For this review, take the finished solid that the model builds, in its own axes (mm). Face numbers are marked on the shaded views. A direction names the side the tool comes from. Give positions to 0.01 mm unless a question says otherwise; leave off trailing zeros. Write each loop counter-clockwise with the first axis right and the second up, starting at its lowest first coordinate (ties: lowest second). Pieces come first, ordered by that corner, then holes.
1) We need section B-B on x = 21.5. Give the boundary of the cut face in (y, z), and give its area (3 significant figures).
2) For P1, Ø1.5, axis at x = 5, z = 4, coming from the -Y side; P2, Ø2, axis at x = 21.5, z = 17.5, coming from the +Y side; P3, Ø7.5, axis at y = -0.5, z = 25, coming from the -X side; P4, Ø2.5, axis at x = 22.5, y = 2.5, coming from the +Z side, all flat-tipped, find the tip position at first contact; note any pin that passes through.
3) Machinability: for the marked faces 1 and 2, which of the approach directions +Z, -Z, +X, -X, +Y, -Y give a long, thin tool a straight path to every point of the face, cutting with its end or side? Answer none if there is none.
4) We need section A-A on x = 0. Give the boundary of the cut face in (y, z).
5) Draft analysis for pull direction X (two halves, no side actions). For the marked faces 3, 4 and 5, state which applies: pulls with the +X half, pulls with the -X half, needs draft (parallel to the pull), parting line crosses it, or undercut.
6) We need section C-C on z = 32.5. Give the boundary of the cut face in (x, y), and give its area (3 significant figures).
7) We need section D-D on z = 17.5. Give the number of separate pieces and of enclosed holes in the cut face, and give its area (3 significant figures).
8) Wall thickness on line 1 along X through (y, z) = (1.5, 18); line 2 along X through (y, z) = (6.75, 17.5); line 3 along Z through (x, y) = (21.5, 1.65): over which ranges is each line inside the solid? List them lowest first.
from build123d import *

# Parameters (mm, degrees)
BOSS_EXTRUDE1_DEPTH  = 35
SKETCH3_W            = 7
SKETCH3_H            = 7
BOSS_EXTRUDE2_DEPTH  = 3
FILLET1_R            = 2
FILLET2_R            = 0.5
M2_CLEARANCE_HOLE1_D = 2.6
FILLET3_R            = 0.5
FILLET4_R            = 2
FILLET5_R            = 10
SKETCH8_W            = 20
SKETCH8_H            = 2
BOSS_EXTRUDE4_DEPTH  = 20
M4_CLEARANCE_HOLE1_D = 4.8
FILLET6_R            = 3
FILLET7_R            = 1


with BuildPart() as part:
    # Sketch1 → Boss-Extrude1 (new body)
    with BuildSketch(Plane.XY):
        with BuildLine():
            Line((13.479150567, 0.75), (17.5, 0.75))
            Line((17.5, 0.75), (17.5, 17.5))
            Line((17.5, 17.5), (-17.5, 17.5))
            Line((-17.5, 17.5), (-17.5, -17.5))
            Line((-17.5, -17.5), (17.5, -17.5))
            Line((17.5, -17.5), (17.5, -0.75))
            Line((17.5, -0.75), (13.479150567, -0.75))
            ThreePointArc((13.479150567, -0.75), (-13.5, 0), (13.479150567, 0.75))
        make_face()
    extrude(amount=BOSS_EXTRUDE1_DEPTH)

    # Sketch3 → Boss-Extrude2 (add)
    with BuildSketch(Plane.XZ.offset(-0.75)):
        with Locations((21, 17.5)):
            Rectangle(SKETCH3_W, SKETCH3_H)
    boss_extrude2 = extrude(amount=-BOSS_EXTRUDE2_DEPTH)

    # Fillet1
    fillet1_edges = [part.edges().sort_by_distance(p)[0] for p in [
        (17.5, 3.75, 17.5),
    ]]
    fillet(fillet1_edges, radius=FILLET1_R)

    # Fillet2
    fillet2_edges = [part.edges().sort_by_distance(p)[0] for p in [
        (24.5, 3.75, 17.5),
    ]]
    fillet(fillet2_edges, radius=FILLET2_R)

    # M2 Clearance Hole1 (through all)
    with Locations(Plane(origin=(0, 3.75, 0), x_dir=(1, 0, 0), z_dir=(0, 1, 0))):
        with Locations((21.5, -17.5)):
            m2_clearance_hole1 = Hole(M2_CLEARANCE_HOLE1_D / 2)

    # Mirror3: Boss-Extrude2 across plane
    add(boss_extrude2.mirror(Plane.ZX))

    # Mirror5: M2 Clearance Hole1 across plane
    add(m2_clearance_hole1.mirror(Plane.ZX), mode=Mode.SUBTRACT)

    # Fillet3
    fillet3_edges = [part.edges().sort_by_distance(p)[0] for p in [
        (24.5, -3.75, 17.5),
    ]]
    fillet(fillet3_edges, radius=FILLET3_R)

    # Fillet4
    fillet4_edges = [part.edges().sort_by_distance(p)[0] for p in [
        (17.5, -3.75, 17.5),
    ]]
    fillet(fillet4_edges, radius=FILLET4_R)

    # Fillet5
    # the kernel refuses this fillet: 10 mm, written as the material it takes off along each edge
    with BuildSketch(Plane(origin=(-42.5, -17.5, 0), x_dir=(0, 0, 1), z_dir=(1, 0, 0)), Plane(origin=(17.5, -17.5, -25), x_dir=(-1, 0, 0), z_dir=(0, 0, 1)), Plane(origin=(42.5, 17.5, 35), x_dir=(0, -1, 0), z_dir=(-1, 0, 0)), Plane(origin=(42.5, 17.5, 0), x_dir=(0, 0, 1), z_dir=(-1, 0, 0)), Plane(origin=(-42.5, -17.5, 35), x_dir=(0, 1, 0), z_dir=(1, 0, 0))) as fillet5_piece_1:
        with BuildLine():
            CenterArc((FILLET5_R, -FILLET5_R), FILLET5_R, 90, 90)
            Line((0, -FILLET5_R), (0, 0))
            Line((0, 0), (FILLET5_R, 0))
        make_face()
    extrude(amount=85, mode=Mode.SUBTRACT)
    with BuildSketch(Plane(origin=(-17.5, 17.5, -25), x_dir=(0, -1, 0), z_dir=(0, 0, 1)), Plane(origin=(17.5, 17.5, -25), x_dir=(-1, 0, 0), z_dir=(0, 0, 1)), Plane(origin=(-17.5, -17.5, -25), x_dir=(1, 0, 0), z_dir=(0, 0, 1))) as fillet5_piece_2:
        with BuildLine():
            CenterArc((FILLET5_R, FILLET5_R), FILLET5_R, 180, 90)
            Line((0, FILLET5_R), (0, 0))
            Line((0, 0), (FILLET5_R, 0))
        make_face()
    extrude(amount=85, mode=Mode.SUBTRACT)

    # Sketch8 → Boss-Extrude4 (add)
    with BuildSketch(Plane.ZY.offset(17.5)):
        with Locations((17.5, 6.5)):
            Rectangle(SKETCH8_W, SKETCH8_H)
    extrude(amount=BOSS_EXTRUDE4_DEPTH)

    # M4 Clearance Hole1 (through all)
    with Locations(Plane(origin=(0, 7.5, 0), x_dir=(1, 0, 0), z_dir=(0, 1, 0))):
        with Locations((-29.5, -17.5)):
            Hole(M4_CLEARANCE_HOLE1_D / 2)

    # Fillet6
    fillet6_edges = [part.edges().sort_by_distance(p)[0] for p in [
        (-17.5, 5.5, 17.5),
        (-17.5, 7.5, 17.5),
    ]]
    fillet(fillet6_edges, radius=FILLET6_R)

    # Fillet7
    fillet7_edges = [part.edges().sort_by_distance(p)[0] for p in [
        (-37.5, 6.5, 7.5),
        (-37.5, 6.5, 27.5),
    ]]
    fillet(fillet7_edges, radius=FILLET7_R)


solid = part.part
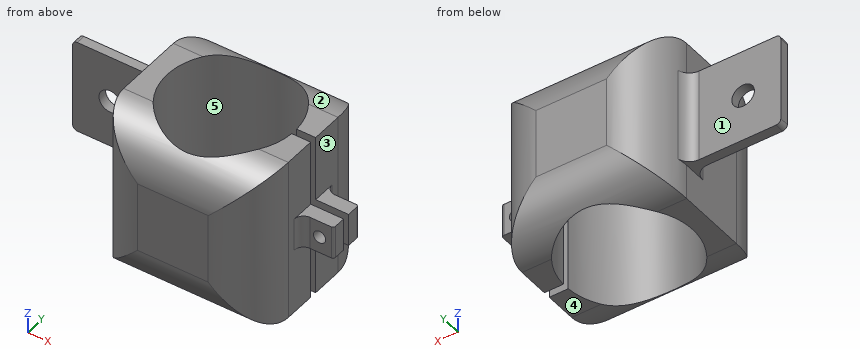
Results list:
1. outline: (-3.75, 14) - (-0.75, 14) - (-0.75, 16.2) - (-3.75, 16.2) - close; (-3.75, 18.8) - (-0.75, 18.8) - (-0.75, 21) - (-3.75, 21) - close; (0.75, 14) - (3.75, 14) - (3.75, 16.2) - (0.75, 16.2) - close; (0.75, 18.8) - (3.75, 18.8) - (3.75, 21) - (0.75, 21) - close
1. area: 26.4 mm2
2. P1: stops at y = -16.01
2. P2: passes through
2. P3: stops at x = -17.6
2. P4: stops at z = 21
3. face 1: +Z, -Z, -X, +Y
3. face 2: +Z, +X, -X, +Y
4. outline: (-17.5, 10) arc R10 ccw to (-13.5, 2) - (-13.5, 33) arc R10 ccw to (-17.5, 25) - close; (13.5, 2) arc R10 ccw to (17.5, 10) - (17.5, 25) arc R10 ccw to (13.5, 33) - close
5. face 3: pulls with the +X half
5. face 4: needs draft
5. face 5: undercut
6. outline: (-17.5, -7.5) arc R10 ccw to (-15, -14.11) - (15, -14.11) arc R10 ccw to (17.5, -7.5) - (17.5, -0.75) - (13.48, -0.75) arc R13.5 cw (long way) to (13.48, 0.75) - (17.5, 0.75) - (17.5, 7.5) arc R10 ccw to (15, 14.11) - (-15, 14.11) arc R10 ccw to (-17.5, 7.5) - close
6. area: 389 mm2
7. separate pieces: 4
7. enclosed holes: 0
7. area: 622 mm2
8. line 1: x = -17.5 to -13.42, 13.42 to 20.3, 22.7 to 24.5
8. line 2: x = -37.5 to -31.9, -27.1 to -11.69, 11.69 to 17.5
8. line 3: z = 14 to 16.2, 18.8 to 21
